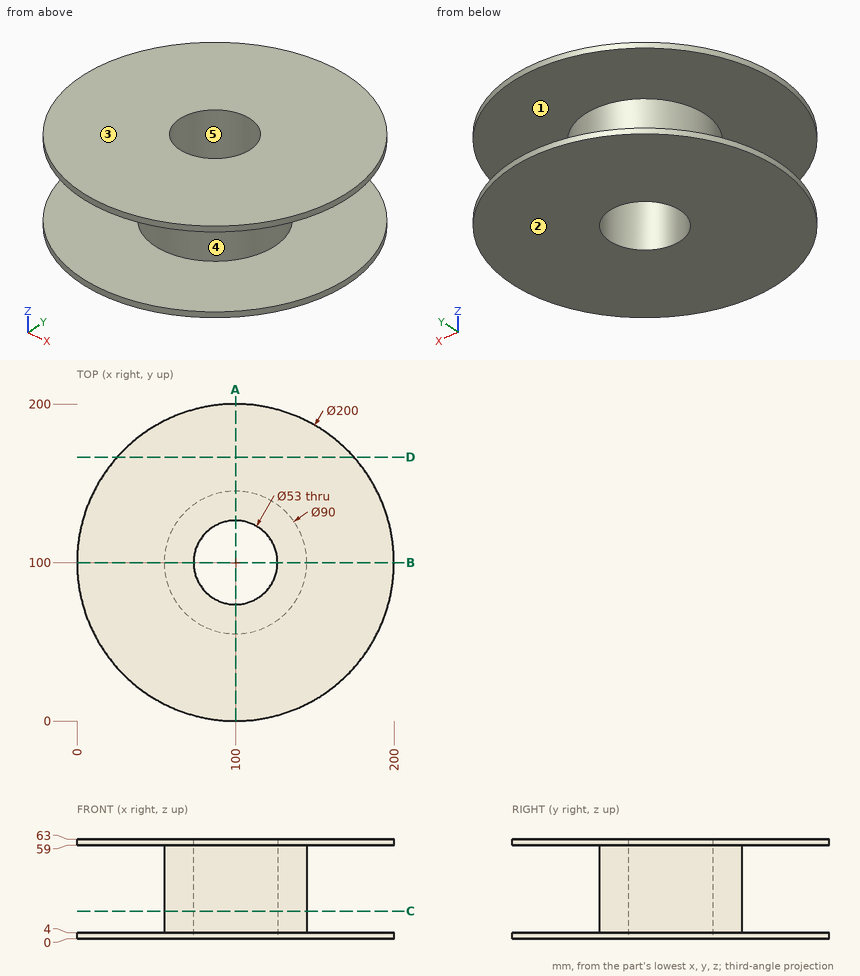
The figure shows three views and two pictorial views of one solid part (mm, origin at its lowest corner). Answer the questions. A direction names the side the tool comes from. Coordinates: 2 decimals unless noted, no trailing zeros. Loops run counter-clockwise (first coordinate to the right, second up) from the corner with the lowest first, then second, coordinate; pieces in that order, holes last. Notation, with made-up numbers: M -23,-15 L -13,-15 A22 cw -13,-8 Z; hole C -29,82.5 d5. An arc over 180 degrees is marked long. Use CSV: the item, a comma, the result in double quotes. Start each with the question number.
(1) Find section A-A, the plane x = 100. Give the vertices of the cut face in (y, z), then the cut area to 3 significant figures.
(2) For the marked faces 1 and 2, determine the directions among +Z, -Z, +X, -X, +Y, -Y from which every point of the face is accessible in a straight line to the end or side of a thin tool.
(3) Consider line 1 (Z direction, x = 42.5, y = 133.5); line 2 (Y direction, x = 100, z = 34); line 3 (X direction, y = 102.5, z = 52.5). Determine where each line is inside the solid, lowest interval first.
(4) Find section D-D, the plane y = 166.5. Give the vertices of the cut face in (x, z), then the cut area to 3 significant figures.
(5) Given pin 1 Ø6 at (y, z) = (117, 38) entering from +X; pin 2 Ø10 at (x, z) = (66, 44.5) entering from +Y; pin 3 Ø2 at (y, z) = (66.5, 20) entering from +X, each flat-ended and moving along its own axis, determine where each tip first touches the part or whether it passes through.
(6) For a pull along Y with two mould halves and no side action, classify the marked faces 3, 4 and 5 as +Y half, -Y half, draft (parallel to the pull), parting line (faces both ways), or undercut.
(7) Find section C-C, the plane z = 17.5. Give the vertices of the cut face in (x, y).
Recorded:
1,outline,"M 0,0 L 73.5,0 L 73.5,63 L 0,63 L 0,59 L 55,59 L 55,4 L 0,4 Z; M 126.5,0 L 200,0 L 200,4 L 145,4 L 145,59 L 200,59 L 200,63 L 126.5,63 Z"
1,area,"3,210 mm^2"
2,face 1,"none"
2,face 2,"-Z, +X, -X, +Y, -Y"
3,line 1,"z = 0 to 4, 59 to 63"
3,line 2,"y = 55 to 73.5, 126.5 to 145"
3,line 3,"x = 55.07 to 73.62, 126.38 to 144.93"
4,outline,"M 25.32,0 L 174.68,0 L 174.68,4 L 25.32,4 Z; M 25.32,59 L 174.68,59 L 174.68,63 L 25.32,63 Z"
4,area,"1,190 mm^2"
5,pin 1,"stops at x = 142.77"
5,pin 2,"stops at y = 134.41"
5,pin 3,"stops at x = 131.12"
6,face 3,"draft"
6,face 4,"parting line"
6,face 5,"undercut"
7,outline,"C 100,100 d90; hole C 100,100 d53"
